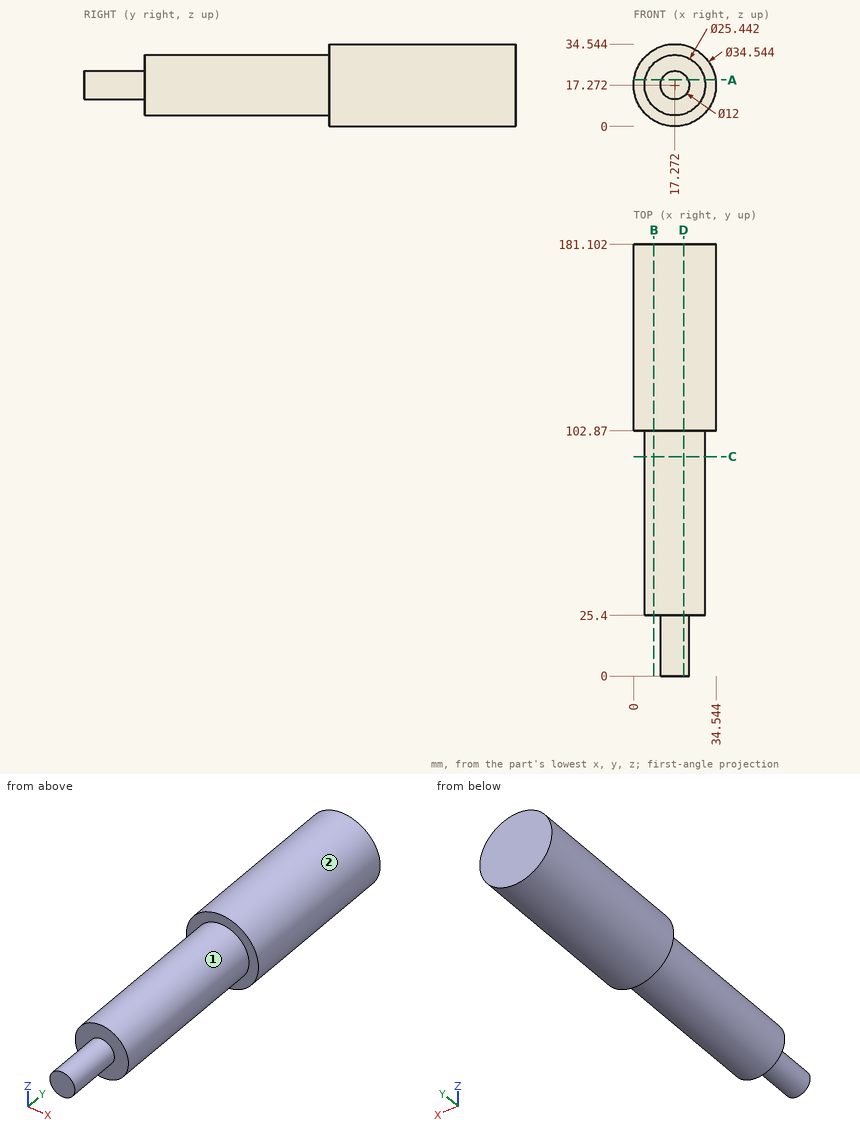
Part print with two shaded views. Sizes in mm from the minimum x, y, z corner. A direction names the side the tool comes from. Round coordinates to 2 decimals unless told otherwise and drop trailing zeros. Loops run counter-clockwise (first coordinate to the right, second up) from the corner with the lowest first, then second, coordinate; pieces in that order, holes last. Notation, with made-up numbers: (13.5, 66) - (28.5, 66) arc R27 cw to (28.5, 88) - close; hole circle Ø7 at (84.25, -37). An arc over 180 degrees is marked (long way). Put each result on its own line as item: value.
1. Slice it at A-A on z = 19.5. List the corners of the cut face in (x, y), and give its area (3 significant figures).
Geometry check:
outline: (0.14, 102.87) - (4.75, 102.87) - (4.75, 25.4) - (11.7, 25.4) - (11.7, 0) - (22.84, 0) - (22.84, 25.4) - (29.8, 25.4) - (29.8, 102.87) - (34.4, 102.87) - (34.4, 181.1) - (0.14, 181.1) - close
area: 4,900 mm²
2. Slice it at B-B on x = 8.5. List the corners of the cut face in (y, z).
Geometry check:
outline: (25.4, 8.06) - (102.87, 8.06) - (102.87, 2.39) - (181.1, 2.39) - (181.1, 32.15) - (102.87, 32.15) - (102.87, 26.48) - (25.4, 26.48) - close
3. Wall check: line 1 (Y direction, x = 32, z = 20); line 2 (Y direction, x = 17, z = 24.5); line 3 (X direction, y = 164.5, z = 10). Give the ranges that are in metal, low to high.
Geometry check:
line 1: 102.87 to 181.1
line 2: 25.4 to 181.1
line 3: 1.61 to 32.94
4. Slice it at C-C on y = 92. List the corners of the cut face in (x, z), and give its area (3 significant figures).
Geometry check:
outline: circle Ø25.44 at (17.27, 17.27)
area: 508 mm²
5. Slice it at D-D on x = 21. List the corners of the cut face in (y, z), and give its area (3 significant figures).
Geometry check:
outline: (0, 12.57) - (25.4, 12.57) - (25.4, 5.11) - (102.87, 5.11) - (102.87, 0.41) - (181.1, 0.41) - (181.1, 34.14) - (102.87, 34.14) - (102.87, 29.43) - (25.4, 29.43) - (25.4, 21.97) - (0, 21.97) - close
area: 4,760 mm²
6. 3-axis set-ups, long thin cutter, end or side, ignore diameter. For the marked faces 1 and 2: which of +Z, -Z, +X, -X, +Y, -Y reach the whole face in a straight line?
Geometry check:
face 1: -Y
face 2: +Y, -Y
7. Pin check, flat tips, straight feed: P1, Ø3, axis at x = 3.5, z = 17.5, coming from the -Y side; P2, Ø1, axis at y = 95, z = 15, coming from the -X side (3 decimals); P3, Ø1, axis at x = 9, y = 40, coming from the -Z side. Stop position of each tip, or through.
Geometry check:
P1: y = 25.4
P2: x = 4.675
P3: z = 7.2
